```python
from build123d import *

# Parameters (mm, degrees)
F0_R     = 12.5
F0_R_2   = 10
F1_DEPTH = 3
F2_R     = 1


with BuildPart() as f1:
    # F0 (on Right) → F1 (new body, symmetric)
    with BuildSketch(Plane.YZ):
        Circle(F0_R)
        Circle(F0_R_2, mode=Mode.SUBTRACT)
    extrude(amount=F1_DEPTH, both=True)

    # F2
    f2_edges = [f1.edges().sort_by_distance(p)[0] for p in [
        (3, -12.5, 0),
        (3, -10, 0),
        (-3, -10, 0),
        (-3, -12.5, 0),
    ]]
    fillet(f2_edges, radius=F2_R)


solid = f1.part
```
Input: part model. Units: mm. Frame: model coordinates. Round coordinates to 2 decimals unless told otherwise and drop trailing zeros. Write each loop counter-clockwise with the first axis right and the second up, starting at its lowest first coordinate (ties: lowest second). Pieces come first, ordered by that corner, then holes. Notation, with made-up numbers: (54.25, 34) -> (88.25, 34) arc R5 ccw to (88.25, 39) -> close; hole circle Ø4 at (85.5, 24.25). An arc over 180 degrees is marked (long way). Answer as CSV lines item,"result".
1. Section D-D (x = 2.5). Return the cut outline in (y, z).
Geometry says:
outline,"circle Ø24.73 at (0, 0); hole circle Ø20.27 at (0, 0)"
2. Mould query, pull axis Y, two halves, no side actions, for faces 1 (the cylindrical face through (-0.03, -2.17, -9.76)), 2 (the cylindrical face through (0.028, 11.923, 3.755)). Classes: +Y half, -Y half, draft (parallel to the pull), parting line (faces both ways), or undercut.
Geometry says:
face 1,"undercut"
face 2,"parting line"
3. Section C-C (x = -0.2). Return the cut outline in (y, z).
Geometry says:
outline,"circle Ø25 at (0, 0); hole circle Ø20 at (0, 0)"
4. Ray query, L1, parallel to Z at x = 0.85, y = 0; L2, parallel to Z at x = -2, y = 4.75; L3, parallel to Y at x = 2.75, z = 7.75. Return the intervals inside material, ascending. Write a range as [from, to].
Geometry says:
L1,"z = [-12.5, -10], [10, 12.5]"
L2,"z = [-11.56, -8.8], [8.8, 11.56]"
L3,"y = [-9.37, -6.84], [6.84, 9.37]"
5. Section A-A (y = 0). Return the cut outline in (x, z).
Geometry says:
outline,"(-3, -11.5) arc R1 ccw to (-2, -12.5) -> (2, -12.5) arc R1 ccw to (3, -11.5) -> (3, -11) arc R1 ccw to (2, -10) -> (-2, -10) arc R1 ccw to (-3, -11) -> close; (-3, 11) arc R1 ccw to (-2, 10) -> (2, 10) arc R1 ccw to (3, 11) -> (3, 11.5) arc R1 ccw to (2, 12.5) -> (-2, 12.5) arc R1 ccw to (-3, 11.5) -> close"
